Could you check a few things on this model? Use its own coordinates, in mm. A direction names the side the tool comes from. Coordinates: 2 decimals unless noted, no trailing zeros. Loops run counter-clockwise (first coordinate to the right, second up) from the corner with the lowest first, then second, coordinate; pieces in that order, holes last.
Autodesk Inventor part; units mm, degrees
ref_plane "YZ Plane" through (0, 0, 0) normal (1, 0, 0) x (0, 1, 0)
ref_plane "XZ Plane" through (0, 0, 0) normal (0, 1, 0) x (-1, 0, 0)
ref_plane "XY Plane" through (0, 0, 0) normal (0, 0, 1) x (1, 0, 0)
sketch "Boceto1" plane through (0, 0, 0) normal (0, 0, 1) x (1, 0, 0)
  line L0 (-39.5, -28) -> (39.5, -28)
  line L1 (42.5, -25) -> (42.5, 25)
  line L2 (39.5, 28) -> (-39.5, 28)
  line L3 (-42.5, 25) -> (-42.5, -25)
  line L4 (-42.5, -28) -> (42.5, 28) construction
  line L5 (42.5, -28) -> (-42.5, 28) construction
  arc A0 (-39.5, 28) -> (-42.5, 25) centre (-39.5, 25) ccw
  arc A1 (42.5, 25) -> (39.5, 28) centre (39.5, 25) ccw
  arc A2 (39.5, -28) -> (42.5, -25) centre (39.5, -25) ccw
  arc A3 (-42.5, -25) -> (-39.5, -28) centre (-39.5, -25) ccw
  circle A4 centre (-39.5, 25) radius 1.375
  circle A5 centre (-39.5, -25) radius 1.375
  circle A6 centre (18.5, -25) radius 1.375
  circle A7 centre (18.5, 25) radius 1.375
  point P0 (0, 0)
  dimension "d0" = 85
  dimension "d1" = 56
  dimension "d2" = 3
  dimension "d3" = 2.75
  dimension "d4" = 2.75
  dimension "d5" = 2.75
  dimension "d6" = 2.75
  dimension "d7" = 58
extrude "Extrusión1" add sketch "Boceto1" along normal blind 2
sketch "Boceto2" plane through (0, 0, 2) normal (0, 0, 1) x (1, 0, 0)
  line L0 (26.5, -6.5) -> (44.5, -6.5)
  line L1 (44.5, -6.5) -> (44.5, 8.5)
  line L2 (44.5, 8.5) -> (26.5, 8.5)
  line L3 (26.5, 8.5) -> (26.5, -6.5)
  line L4 (26.5, -6.5) -> (44.5, 8.5) construction
  line L5 (44.5, -6.5) -> (26.5, 8.5) construction
  line L6 (-39.5, -28) -> (39.5, -28)
  line L7 (22.5, -25.75) -> (44.5, -25.75)
  line L8 (44.5, -25.75) -> (44.5, -9.75)
  line L9 (44.5, -9.75) -> (22.5, -9.75)
  line L10 (22.5, -9.75) -> (22.5, -25.75)
  line L11 (22.5, -25.75) -> (44.5, -9.75) construction
  line L12 (44.5, -25.75) -> (22.5, -9.75) construction
  line L13 (-18, -29) -> (-3, -29)
  line L14 (-3, -29) -> (-3, -18)
  line L15 (-3, -18) -> (-18, -18)
  line L16 (-18, -18) -> (-18, -29)
  line L17 (-18, -29) -> (-3, -18) construction
  line L18 (-3, -29) -> (-18, -18) construction
  line L19 (-42.5, 25) -> (-42.5, -25)
  line L20 (8, -16) -> (16, -16)
  line L21 (16, -16) -> (16, -31)
  line L22 (16, -31) -> (8, -31)
  line L23 (8, -31) -> (8, -16)
  line L24 (8, -16) -> (16, -31) construction
  line L25 (16, -16) -> (8, -31) construction
  line L26 (-36.5, -29) -> (-27.5, -29)
  line L27 (-27.5, -29) -> (-27.5, -24)
  line L28 (-27.5, -24) -> (-36.5, -24)
  line L29 (-36.5, -24) -> (-36.5, -29)
  line L30 (-36.5, -29) -> (-27.5, -24) construction
  line L31 (-27.5, -29) -> (-36.5, -24) construction
  line L32 (26.5, 11.5) -> (44.5, 11.5)
  line L33 (44.5, 11.5) -> (44.5, 26.5)
  line L34 (44.5, 26.5) -> (26.5, 26.5)
  line L35 (26.5, 26.5) -> (26.5, 11.5)
  line L36 (26.5, 11.5) -> (44.5, 26.5) construction
  line L37 (44.5, 11.5) -> (26.5, 26.5) construction
  line L38 (42.5, -25) -> (42.5, 25)
  point P0 (0, 0)
  point P1 (35.5, 1)
  point P2 (33.5, -17.75)
  point P3 (-10.5, -23.5)
  point P4 (12, -23.5)
  point P5 (-32, -26.5)
  point P6 (35.5, 19)
  dimension "d11" = 15
  dimension "d15" = 29
  dimension "d18" = 22
  dimension "d19" = 16
  dimension "d20" = 10.25
  dimension "d22" = 15
  dimension "d23" = 11
  dimension "d24" = 1
  dimension "d25" = 32
  dimension "d26" = 8
  dimension "d27" = 15
  dimension "d28" = 3
  dimension "d29" = 54.5
  dimension "d30" = 9
  dimension "d31" = 5
  dimension "d33" = 1
  dimension "d34" = 10.5
  dimension "d45" = 15
  dimension "d46" = 2
  dimension "d47" = 47
extrude "Extrusión3" add sketch "Boceto2" along normal blind 13.5 contours L9 L8 L7 L10
extrude "Extrusión4" add sketch "Boceto2" along normal blind 6 contours L23 L20 L21 L6 | L6 L21 L22 L23
extrude "Extrusión5" add sketch "Boceto2" along normal blind 6.5 contours L16 L15 L14 L6 | L6 L14 L13 L16
extrude "Extrusión6" add sketch "Boceto2" along normal blind 3 contours L29 L28 L27 L6 | L6 L27 L26 L29
extrude "Extrusión7" add sketch "Boceto2" along normal blind 16 contours L3 L2 L38 L0 | L32 L35 L34 L33 | L38 L2 L1 L0
properties part number "RasPi3B+"
(1) Which directions (+Z, -Z, +X, -X, +Y, -Y) give clear straight access to the entire face, cutting with the end or side of a thin tool? Please do faces 4 (the face through (12, -16, 5)), 5 (the face through (36, 8.5, 10)), 6 (the face through (42.5, 0, 1)), 7 (the face through (-32, -29, 3)).
Answers:
face 4: +Z, -X, +Y
face 5: +Z, +X, -X
face 6: -Z, +X, +Y, -Y
face 7: +Z, -Z, -X, -Y
(2) Imagine slicing it at C-C, the plane y = 4. Write out the boundary of the cut face in (x, z), and give its area (3 significant figures).
Answers:
outline: (-42.5, 0) - (42.5, 0) - (42.5, 2) - (44.5, 2) - (44.5, 18) - (26.5, 18) - (26.5, 2) - (-42.5, 2) - close
area: 458 mm2
(3) We'd pull the mould along X, two halves only. Please class faces 1 (the face through (17.487, -25.929, 0.986)), 2 (the face through (-1, -28, 1)), 3 (the face through (44.5, 1, 10)): +X half, -X half, draft (parallel to the pull), parting line (faces both ways), or undercut.
Answers:
face 1: undercut
face 2: draft
face 3: +X half
(4) For pin 1 (5 mm diameter, centred on x = 15.5, y = 2.5, fed in from +Z); pin 2 (5 mm diameter, centred on x = 29.5, y = -18, fed in from +Z); pin 3 (7 mm diameter, centred on x = -13, z = 6, fed in from -Y); pin 4 (12 mm diameter, centred on x = -25.5, y = -4.5, fed in from -Z), each with a flat end and sliding along its axis, tell me the tip position at first contact or that it passes through.
Answers:
pin 1: stops at z = 2
pin 2: stops at z = 15.5
pin 3: stops at y = -29
pin 4: stops at z = 0
(5) Imagine slicing it at B-B, the plane z = 14.5. Write out the boundary of the cut face in (x, y), and give its area (3 significant figures).
Answers:
outline: (22.5, -25.75) - (44.5, -25.75) - (44.5, -9.75) - (22.5, -9.75) - close; (26.5, -6.5) - (44.5, -6.5) - (44.5, 8.5) - (26.5, 8.5) - close; (26.5, 11.5) - (44.5, 11.5) - (44.5, 26.5) - (26.5, 26.5) - close
area: 892 mm2
(6) Imagine slicing it at D-D, the plane x = 34. Write out the boundary of the cut face in (y, z), and give its area (3 significant figures).
Answers:
outline: (-28, 0) - (28, 0) - (28, 2) - (26.5, 2) - (26.5, 18) - (11.5, 18) - (11.5, 2) - (8.5, 2) - (8.5, 18) - (-6.5, 18) - (-6.5, 2) - (-9.75, 2) - (-9.75, 15.5) - (-25.75, 15.5) - (-25.75, 2) - (-28, 2) - close
area: 808 mm2
(7) I need wall thicknesses on probe 1 along Y at (x, z) = (18.5, 1.5) (3 decimals); probe 2 along Y at (x, z) = (33, 11.25); probe 3 along X at (y, z) = (-21, 6.25). Which ranges of each line are inside material? Lowest first, please.
Answers:
probe 1: y = -28 to -26.375, -23.625 to 23.625, 26.375 to 28
probe 2: y = -25.75 to -9.75, -6.5 to 8.5, 11.5 to 26.5
probe 3: x = -18 to -3, 8 to 16, 22.5 to 44.5
(8) Imagine slicing it at A-A, the plane z = 6. Write out the boundary of the cut face in (x, y).
Answers:
outline: (-18, -29) - (-3, -29) - (-3, -18) - (-18, -18) - close; (8, -31) - (16, -31) - (16, -16) - (8, -16) - close; (22.5, -25.75) - (44.5, -25.75) - (44.5, -9.75) - (22.5, -9.75) - close; (26.5, -6.5) - (44.5, -6.5) - (44.5, 8.5) - (26.5, 8.5) - close; (26.5, 11.5) - (44.5, 11.5) - (44.5, 26.5) - (26.5, 26.5) - close
